Could you check a few things on this model? Use its own coordinates, in mm. Face numbers are marked on the shaded views. A direction names the side the tool comes from. Round coordinates to 2 decimals unless told otherwise and drop trailing zeros. Loops run counter-clockwise (first coordinate to the right, second up) from the corner with the lowest first, then second, coordinate; pieces in that order, holes last. Notation, with made-up numbers: (-5.5, 60.25) -> (1.5, 60.25) arc R35 cw to (1.5, 97.25) -> close; hole circle Ø5 at (62, 81). An arc over 180 degrees is marked (long way). Write each question's results on one line, items separated by ' | '. Start each with the question number.
1) We'd pull the mould along X, two halves only. Please class the marked faces 3 and 4: pulls with the +X half, pulls with the -X half, needs draft (parallel to the pull), parting line crosses it, or undercut.
2) Which directions (+Z, -Z, +X, -X, +Y, -Y) give clear straight access to the entire face, cutting with the end or side of a thin tool? Please do the marked faces 1 and 2.
3) Imagine slicing it at A-A, the plane y = 22.25. List the corners of the cut face in (x, z) for me, plus the area to 3 significant figures.
4) Imagine slicing it at C-C, the plane z = 2.9. List the corners of the cut face in (x, y) for me.
5) Imagine slicing it at B-B, the plane x = 11. List the corners of the cut face in (y, z) for me, plus the area to 3 significant figures.
6) If I drill on probe 1 along X at (y, z) = (19.25, 0.35); probe 2 along Y at (x, z) = (4, 2.2), over which ranges is the centre line in solid material (lowest first)?
from build123d import *

# Parameters (mm, degrees)
F0_W     = 40
F0_H     = 25
F0_W_2   = 9.283639
F0_H_2   = 8.530912
F1_DEPTH = 5


with BuildPart() as f1:
    # F0 (on Top) → F1 (new body)
    with BuildSketch(Plane.XY):
        with Locations((20, 12.5)):
            Rectangle(F0_W, F0_H)
        with Locations((6.75697, 6.363504)):
            Rectangle(F0_W_2, F0_H_2, mode=Mode.SUBTRACT)
        with Locations((19.75697, 6.363504)):
            Rectangle(F0_W_2, F0_H_2, mode=Mode.SUBTRACT)
        with Locations((32.75697, 6.363504)):
            Rectangle(F0_W_2, F0_H_2, mode=Mode.SUBTRACT)
        with Locations((6.75697, 18.636496)):
            Rectangle(F0_W_2, F0_H_2, mode=Mode.SUBTRACT)
        with Locations((19.75697, 18.636496)):
            Rectangle(F0_W_2, F0_H_2, mode=Mode.SUBTRACT)
        with Locations((32.75697, 18.636496)):
            Rectangle(F0_W_2, F0_H_2, mode=Mode.SUBTRACT)
    extrude(amount=F1_DEPTH)


solid = f1.part
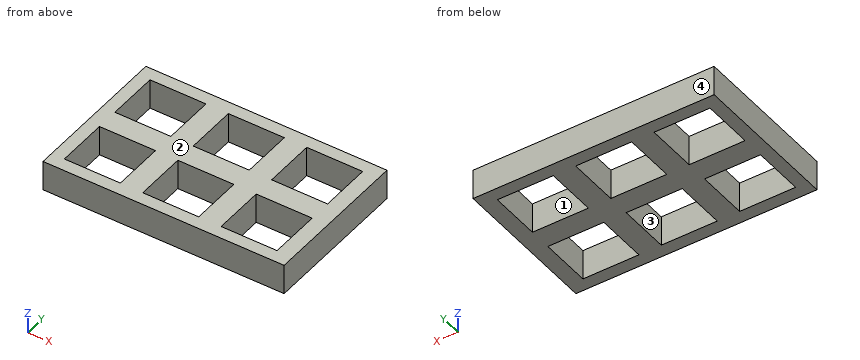
Checked values:
1) face 3: undercut | face 4: needs draft
2) face 1: +Z, -Z | face 2: +Z, +X, -X, +Y, -Y
3) outline: (0, 0) -> (2.12, 0) -> (2.12, 5) -> (0, 5) -> close; (11.4, 0) -> (15.12, 0) -> (15.12, 5) -> (11.4, 5) -> close; (24.4, 0) -> (28.12, 0) -> (28.12, 5) -> (24.4, 5) -> close; (37.4, 0) -> (40, 0) -> (40, 5) -> (37.4, 5) -> close | area: 60.7 mm^2
4) outline: (0, 0) -> (40, 0) -> (40, 25) -> (0, 25) -> close; hole (2.12, 2.1) -> (11.4, 2.1) -> (11.4, 10.63) -> (2.12, 10.63) -> close; hole (2.12, 14.37) -> (11.4, 14.37) -> (11.4, 22.9) -> (2.12, 22.9) -> close; hole (15.12, 2.1) -> (24.4, 2.1) -> (24.4, 10.63) -> (15.12, 10.63) -> close; hole (15.12, 14.37) -> (24.4, 14.37) -> (24.4, 22.9) -> (15.12, 22.9) -> close; hole (28.12, 2.1) -> (37.4, 2.1) -> (37.4, 10.63) -> (28.12, 10.63) -> close; hole (28.12, 14.37) -> (37.4, 14.37) -> (37.4, 22.9) -> (28.12, 22.9) -> close
5) outline: (0, 0) -> (2.1, 0) -> (2.1, 5) -> (0, 5) -> close; (10.63, 0) -> (14.37, 0) -> (14.37, 5) -> (10.63, 5) -> close; (22.9, 0) -> (25, 0) -> (25, 5) -> (22.9, 5) -> close | area: 39.7 mm^2
6) probe 1: 0 to 2.12, 11.4 to 15.12, 24.4 to 28.12, 37.4 to 40 | probe 2: 0 to 2.1, 10.63 to 14.37, 22.9 to 25
